The model under review builds one solid part; all positions refer to its coordinate system, in mm. Face numbers are marked on the shaded views. A direction names the side the tool comes from. Round coordinates to 2 decimals unless told otherwise and drop trailing zeros. Order: outer loops, then holes, each group sorted by start corner. A loop starts at its lowest first (then second) coordinate and runs counter-clockwise, first axis right, second up. Notation, with made-up numbers: (4, -19) - (22, -19) arc R29 ccw to (22, 17) - close; hole circle Ø10 at (59.25, -22.75). An arc over 180 degrees is marked (long way). One line per question, with ' | ' between items. Start each with the question number.
Item 1: For L1, parallel to X at y = 32, z = 4.5; L2, parallel to Y at x = 40, z = 13; L3, parallel to Y at x = 83, z = -23, list the stretches that pass through material, from the lowest coordinate up. Write a range as [from, to].
Item 2: Add section C-C on y = 50. State the section outline as (x, z) points, and give its area (3 significant figures).
Item 3: Tool access review of the marked faces 1, 2, 3 and 4: name each direction out of +Z, -Z, +X, -X, +Y, -Y from which nothing blocks a thin tool from reaching the whole face with its end or side.
Item 4: Add section B-B on z = 7. State the section outline as (x, y) points.
Item 5: Add section A-A on x = 85. State the section outline as (y, z) points, and give its area (3 significant figures).
Item 6: Add section D-D on x = 40. State the section outline as (y, z) points.
Item 7: Draft analysis for pull direction Y (two halves, no side actions). For the marked faces 5, 6 and 7, state which applies: +Y half, -Y half, draft (parallel to the pull), parting line (faces both ways), or undercut.
Item 8: Insertion check: pin 1 Ø4.5 at (x, z) = (2.5, 4.5) entering from -Y; pin 2 Ø10.5 at (y, z) = (40, -15) entering from -X; pin 3 Ø5 at (x, z) = (84.5, -17.5) entering from -Y. Each pin has a flat end and moves straight along its axis. Give the tip position at first contact, or say it passes through.
from build123d import *

# Parameters (mm, degrees)
SKETCH1_W           = 80
SKETCH1_H           = 80
SKETCH1_R           = 32
BOSS_EXTRUDE1_DEPTH = 15
BOSS_EXTRUDE2_START = -2.8
SKETCH2_R           = 32
SKETCH2_R_2         = 27.5
BOSS_EXTRUDE2_DEPTH = 2.8
FILLET1_R           = 10
SKETCH4_W           = 40
SKETCH4_H           = 60
BOSS_EXTRUDE3_DEPTH = 10
SKETCH10_R          = 2.5
CUT_EXTRUDE2_DEPTH  = 127.885775404
BOSS_EXTRUDE7_DEPTH = 10
CUT_EXTRUDE3_DEPTH  = 10
SKETCH13_R          = 1.5
CUT_EXTRUDE5_DEPTH  = 30
SKETCH14_R          = 15
CUT_EXTRUDE6_DEPTH  = 2
SKETCH16_W          = 60.967741935
SKETCH16_H          = 31.937806786
CUT_EXTRUDE10_DEPTH = 12
SKETCH17_W          = 80
SKETCH17_H          = 10
CUT_EXTRUDE11_DEPTH = 12
SKETCH18_R          = 2
CUT_EXTRUDE12_DEPTH = 20
SKETCH21_W          = 9.032258065
SKETCH21_H          = 31.937806786
SKETCH21_W_2        = 70.967741935
CUT_EXTRUDE14_DEPTH = 12


with BuildPart() as part:
    # Sketch1 → Boss-Extrude1 (new body)
    with BuildSketch(Plane.XY):
        with Locations((40, 40)):
            Rectangle(SKETCH1_W, SKETCH1_H)
        with Locations((40, 40)):
            Circle(SKETCH1_R, mode=Mode.SUBTRACT)
    extrude(amount=BOSS_EXTRUDE1_DEPTH)

    # Sketch2 → Boss-Extrude2 (add)
    with BuildSketch(Plane.XY.offset(15).offset(BOSS_EXTRUDE2_START)):
        with Locations((40, 40)):
            Circle(SKETCH2_R)
        with Locations((40, 40)):
            Circle(SKETCH2_R_2, mode=Mode.SUBTRACT)
    extrude(amount=BOSS_EXTRUDE2_DEPTH)

    # Fillet1
    fillet1_edges = [part.edges().sort_by_distance(p)[0] for p in [
        (0, 80, 7.5),
        (80, 80, 7.5),
        (80, 0, 7.5),
        (0, 0, 7.5),
    ]]
    fillet(fillet1_edges, radius=FILLET1_R)

    # Sketch4 → Boss-Extrude3 (add)
    with BuildSketch(Plane(origin=(80, 0, 0), x_dir=(0, 0, -1), z_dir=(1, 0, 0))):
        with Locations((5, 40)):
            Rectangle(SKETCH4_W, SKETCH4_H)
    extrude(amount=BOSS_EXTRUDE3_DEPTH)

    # Sketch10 → Cut-Extrude2 (cut, through all)
    with BuildSketch(Plane(origin=(0, 0, -25), x_dir=(-1, 0, 0), z_dir=(0, 0, -1))):
        with Locations(Location((-85, 55, 0), (0, 0, 90))):
            Circle(SKETCH10_R)
        with Locations(Location((-85, 25, 0), (0, 0, 270))):
            Circle(SKETCH10_R)
    extrude(amount=-CUT_EXTRUDE2_DEPTH, mode=Mode.SUBTRACT)

    # Sketch11 → Boss-Extrude7 (add)
    with BuildSketch(Plane(origin=(90, 0, 0), x_dir=(0, 0, -1), z_dir=(1, 0, 0))):
        Polygon((25, 70), (25, 66), (29, 70), align=None)
        Polygon((25, 14), (29, 10), (25, 10), align=None)
    extrude(amount=-BOSS_EXTRUDE7_DEPTH)

    # Sketch12 → Cut-Extrude3 (cut)
    with BuildSketch(Plane(origin=(90, 0, 0), x_dir=(0, 0, -1), z_dir=(1, 0, 0))):
        with BuildLine():
            Line((18.45172909, 42.02127838), (18.45172909, 37.97872162))
            ThreePointArc((18.45172909, 37.97872162), (11, 40), (18.45172909, 42.02127838))
        make_face()
    extrude(amount=-CUT_EXTRUDE3_DEPTH, mode=Mode.SUBTRACT)

    # Sketch13 → Cut-Extrude5 (cut)
    with BuildSketch(Plane(origin=(90, 0, 0), x_dir=(0, 0, -1), z_dir=(1, 0, 0))):
        with Locations((15, 50)):
            Circle(SKETCH13_R)
        with Locations((15, 30)):
            Circle(SKETCH13_R)
        with Locations((5, 40)):
            Circle(SKETCH13_R)
    extrude(amount=-CUT_EXTRUDE5_DEPTH, mode=Mode.SUBTRACT)

    # Sketch14 → Cut-Extrude6 (cut)
    with BuildSketch(Plane(origin=(90, 0, 0), x_dir=(0, 0, -1), z_dir=(1, 0, 0))):
        with Locations((15, 40)):
            Circle(SKETCH14_R)
    extrude(amount=-CUT_EXTRUDE6_DEPTH, mode=Mode.SUBTRACT)

    # Sketch16 → Cut-Extrude10 (cut)
    with BuildSketch(Plane(origin=(0, 0, 0), x_dir=(-1, 0, 0), z_dir=(0, 0, -1))):
        with Locations((-39.516129033, 15.968903393)):
            Rectangle(SKETCH16_W, SKETCH16_H)
    extrude(amount=-CUT_EXTRUDE10_DEPTH, mode=Mode.SUBTRACT)

    # Sketch17 → Cut-Extrude11 (cut)
    with BuildSketch(Plane(origin=(0, 0, 0), x_dir=(-1, 0, 0), z_dir=(0, 0, -1))):
        with Locations((-40, 5)):
            Rectangle(SKETCH17_W, SKETCH17_H)
    extrude(amount=-CUT_EXTRUDE11_DEPTH, mode=Mode.SUBTRACT)

    # Sketch18 → Cut-Extrude12 (cut)
    with BuildSketch(Plane.XZ.offset(-10)):
        with Locations(Location((5, 6, 0), (0, 0, 270))):
            Circle(SKETCH18_R)
        with Locations(Location((75, 6, 0), (0, 0, 270))):
            Circle(SKETCH18_R)
    extrude(amount=-CUT_EXTRUDE12_DEPTH, mode=Mode.SUBTRACT)

    # Sketch21 → Cut-Extrude14 (cut)
    with BuildSketch(Plane(origin=(0, 0, 0), x_dir=(-1, 0, 0), z_dir=(0, 0, -1))):
        with Locations((-4.516129033, 15.968903393)):
            Rectangle(SKETCH21_W, SKETCH21_H)
        with Locations((-44.516129033, 15.968903393)):
            Rectangle(SKETCH21_W_2, SKETCH21_H)
    extrude(amount=-CUT_EXTRUDE14_DEPTH, mode=Mode.SUBTRACT)


solid = part.part
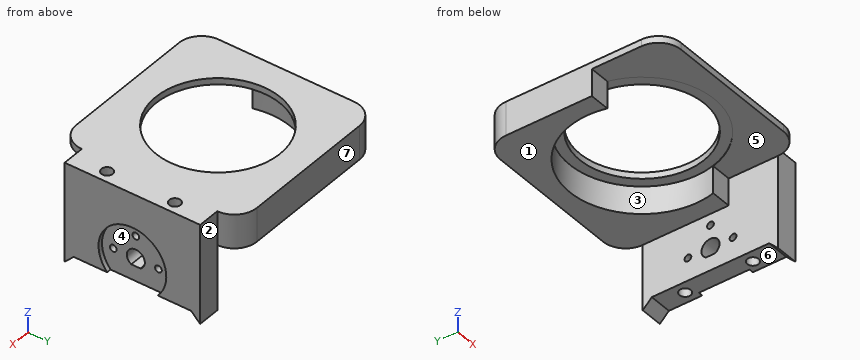
Determined:
1) L1: [0, 9.02], [70.98, 90] | L2: [0, 12.5], [67.5, 80] | L3: [10, 23.5], [26.5, 53.5], [56.5, 70]
2) outline: (0, 0) - (9.6, 0) - (9.6, 12.2) - (14.38, 12.2) - (14.38, 15) - (0, 15) - close; (65.62, 12.2) - (70.4, 12.2) - (70.4, 0) - (80, 0) - (80, -13.5) - (88, -13.5) - (88, -3.82) - (90, -3.82) - (90, 15) - (65.62, 15) - close; (80, -25) - (88, -25) - (88, -16.5) - (80, -16.5) - close | area: 648 mm2
3) face 1: -Z, -X, +Y, -Y | face 2: +Z, -Z, +X, +Y | face 3: -Z | face 4: +X
4) outline: (0, 31.94) - (9.03, 31.94) arc R32 cw (long way) to (70.97, 31.94) - (80, 31.94) - (80, 10) - (90, 10) - (90, 70) - (80, 70) arc R10 ccw to (70, 80) - (10, 80) arc R10 ccw to (0, 70) - close; hole circle Ø5 at (85, 25); hole circle Ø5 at (85, 55)
5) outline: (10, -29) - (14, -25) - (22.5, -25) - (22.5, 15) - (10, 15) - close; (27.5, -25) - (52.5, -25) - (52.5, 15) - (27.5, 15) - close; (57.5, -25) - (66, -25) - (70, -29) - (70, 15) - (57.5, 15) - close; hole circle Ø3 at (30, -15); hole (37.98, -18.45) - (42.02, -18.45) arc R4 ccw (long way) to start; hole circle Ø3 at (40, -5); hole circle Ø3 at (50, -15) | area: 1,950 mm2
6) outline: (0, 12) - (8, 12) - (8, 12.2) - (12.5, 12.2) - (12.5, 15) - (0, 15) - close; (67.5, 12.2) - (72, 12.2) - (72, 0) - (80, 0) - (80, 15) - (67.5, 15) - close
7) face 5: draft | face 6: undercut | face 7: +Y half
8) pin 1: y = 31.94 | pin 2: x = 80 | pin 3: y = 10
